Job drawing, mm, ordinate dimensions from the low corner. One solid piece. A direction names the side the tool comes from. Coordinates: 2 decimals unless noted, no trailing zeros. Loops run counter-clockwise (first coordinate to the right, second up) from the corner with the lowest first, then second, coordinate; pieces in that order, holes last. Notation, with made-up numbers: M 63,2 L 95,2 A26 cw 95,16 Z; hole C 70,25 d7. An arc over 180 degrees is marked long. Write each question's results on one line, items separated by ' | '. Start each with the question number.
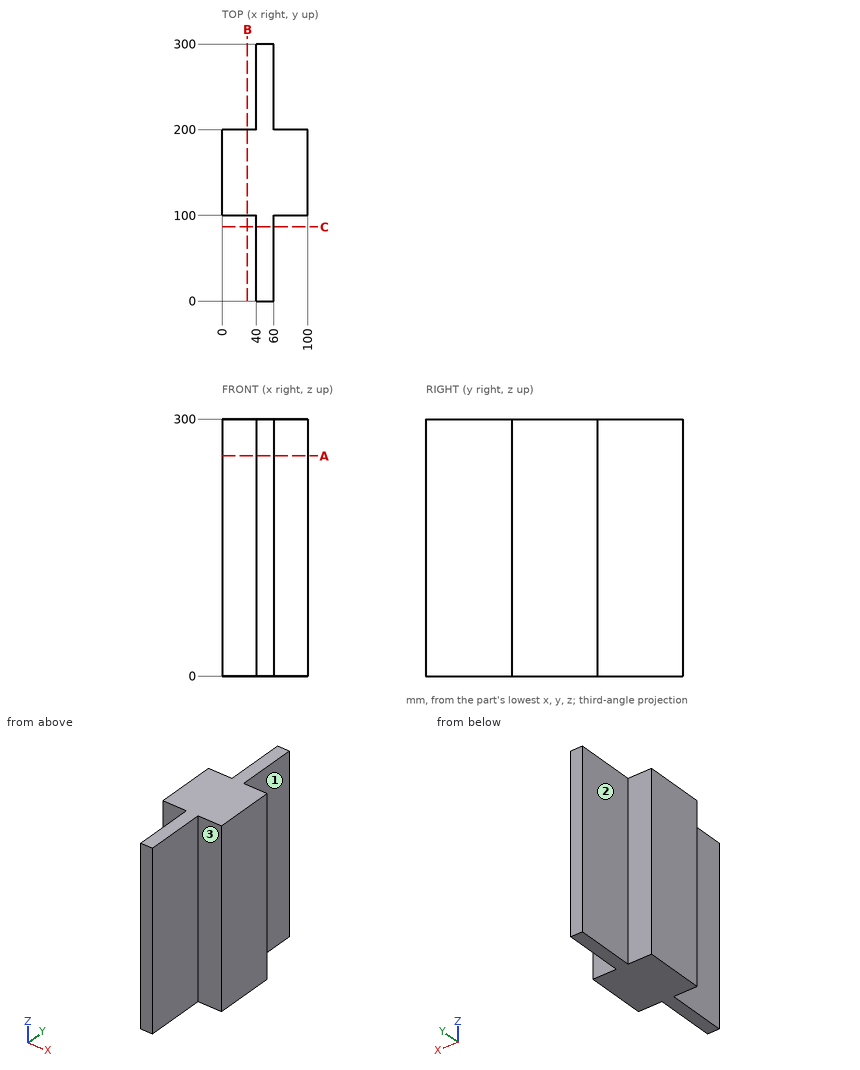
1. Pin check, flat tips, straight feed: pin 1 (8 mm diameter, centred on x = 43, y = 157, fed in from -Z); pin 2 (2 mm diameter, centred on y = 30, z = 259, fed in from +X); pin 3 (12 mm diameter, centred on x = 85, z = 167.5, fed in from +Y); pin 4 (12 mm diameter, centred on y = 59.5, z = 149.5, fed in from -X). Stop position of each tip, or through.
2. Band-saw the part on A-A, the plane z = 257. List the corners of the cut face in (x, y).
3. Which spindle directions (+Z, -Z, +X, -X, +Y, -Y) get a long thin tool onto all of the face, cutting with end or side? Do the marked faces 1, 2 and 3. Say none if no direction does.
4. Band-saw the part on C-C, the plane y = 86.5. List the corners of the cut face in (x, z).
5. Wall check: line 1 along X through (y, z) = (57, 80); line 2 along Y through (x, z) = (33, 288). Give the ranges that are in metal, low to high.
6. Band-saw the part on B-B, the plane x = 29.5. List the corners of the cut face in (y, z), plus the area to 3 significant figures.
Checked values:
1) pin 1: z = 0 | pin 2: x = 60 | pin 3: y = 200 | pin 4: x = 40
2) outline: M 0,100 L 40,100 L 40,0 L 60,0 L 60,100 L 100,100 L 100,200 L 60,200 L 60,300 L 40,300 L 40,200 L 0,200 Z
3) face 1: +Z, -Z, +X, +Y | face 2: +Z, -Z, -X, +Y | face 3: +Z, -Z, +X, -Y
4) outline: M 40,0 L 60,0 L 60,300 L 40,300 Z
5) line 1: 40 to 60 | line 2: 100 to 200
6) outline: M 100,0 L 200,0 L 200,300 L 100,300 Z | area: 30,000 mm²
